from build123d import *

# Parameters (mm, degrees)
SKETCH1_W           = 50.8
SKETCH1_H           = 25.4
SKETCH1_R           = 3.2639
BOSS_EXTRUDE1_DEPTH = 2.38125


with BuildPart() as part:
    # Sketch1 → Boss-Extrude1 (new body, symmetric)
    with BuildSketch(Plane.XY):
        with Locations((25.4, 12.7)):
            Rectangle(SKETCH1_W, SKETCH1_H)
        with Locations((12.7, 12.7)):
            Circle(SKETCH1_R, mode=Mode.SUBTRACT)
        with Locations((38.1, 12.7)):
            Circle(SKETCH1_R, mode=Mode.SUBTRACT)
    extrude(amount=BOSS_EXTRUDE1_DEPTH, both=True)


solid = part.part
Could you check a few things on this model? Use its own coordinates, in mm. Give positions to 0.01 mm unless a question says otherwise; leave off trailing zeros. Order: outer loops, then holes, each group sorted by start corner. A loop starts at its lowest first (then second) coordinate and runs counter-clockwise, first axis right, second up. Notation, with made-up numbers: (-2.5, 23) - (50.5, 23) arc R19 cw to (50.5, 49) - close; hole circle Ø2 at (86, 14). An arc over 180 degrees is marked (long way). Return JSON: item names as keys, results as strings. Group by question number.
Q1. Suppose I cut it at D-D, the plane x = 10.5. Please give me the cut outline in (y, z), and give its area (3 significant figures).
Q2. Please list where these lines run through material, in increasing order: line 1 along Y through (x, z) = (38.1, 0.4); line 2 along Y through (x, z) = (40, 1.5). Write a range as [from, to].
Q3. Suppose I cut it at A-A, the plane x = 38.1. Please give me the cut outline in (y, z).
Q4. Suppose I cut it at B-B, the plane y = 12.7. Please give me the cut outline in (x, z), and give its area (3 significant figures).
Q5. Thinking about a two-plate mould opening in X: for faces 1 (the face through (25, 25.4, 0)), 2 (the face through (0, 13, 0)), 3 (the face through (41.213, 13.68, -0.033)), which applies, pulls with the +X half, pulls with the -X half, needs draft (parallel to the pull), parting line crosses it, or undercut?
Q6. Suppose I cut it at C-C, the plane z = -1.35. Please give me the cut outline in (x, y).
Resolved:
{
 "1": {"outline": "(0, -2.38) - (10.29, -2.38) - (10.29, 2.38) - (0, 2.38) - close; (15.11, -2.38) - (25.4, -2.38) - (25.4, 2.38) - (15.11, 2.38) - close", "area": "98.0 mm2"},
 "2": {"line 1": "y = [0, 9.44], [15.96, 25.4]", "line 2": "y = [0, 10.05], [15.35, 25.4]"},
 "3": {"outline": "(0, -2.38) - (9.44, -2.38) - (9.44, 2.38) - (0, 2.38) - close; (15.96, -2.38) - (25.4, -2.38) - (25.4, 2.38) - (15.96, 2.38) - close"},
 "4": {"outline": "(0, -2.38) - (9.44, -2.38) - (9.44, 2.38) - (0, 2.38) - close; (15.96, -2.38) - (34.84, -2.38) - (34.84, 2.38) - (15.96, 2.38) - close; (41.36, -2.38) - (50.8, -2.38) - (50.8, 2.38) - (41.36, 2.38) - close", "area": "180 mm2"},
 "5": {"face 1": "needs draft", "face 2": "pulls with the -X half", "face 3": "undercut"},
 "6": {"outline": "(0, 0) - (50.8, 0) - (50.8, 25.4) - (0, 25.4) - close; hole circle Ø6.53 at (12.7, 12.7); hole circle Ø6.53 at (38.1, 12.7)"}
}
